Model file for the job. Use its own axes, mm. A direction names the side the tool comes from. Coordinates: 2 decimals unless noted, no trailing zeros. Write each loop counter-clockwise with the first axis right and the second up, starting at its lowest first coordinate (ties: lowest second). Pieces come first, ordered by that corner, then holes. Notation, with made-up numbers: (84, 16.5) - (129, 16.5) arc R22 cw to (129, 45.5) - close; hole circle Ø8 at (36.5, 29). An arc over 180 degrees is marked (long way). Put each result on its own line as item: value. Start each with the question number.
1. Saw through at B-B, the plane y = 0.5. Write the cut outline in (x, z), plus the area to 3 significant figures.
2. Which spindle directions (+Z, -Z, +X, -X, +Y, -Y) get a long thin tool onto all of the face, cutting with end or side? Do faces 3 (the face through (0, 1, 2.5)), 4 (the face through (22, 2, 1)). Say none if no direction does.
3. Drill centre lines: L1, parallel to X at y = 1.5, z = 0; L2, parallel to X at y = 2.7, z = 0; L3, parallel to Y at x = -14, z = -0.3. Where is each one in solid material? Low to high. Write a range as from..to.
4. Pull direction X, two halves, no side cores. Call faces 1 (the face through (21, 1, 0)), 2 (the face through (-24, 3, 0)): released by +X, released by -X, zero draft, split by the parting line, or undercut.
5. Saw through at A-A, the plane z = 0. Write the cut outline in (x, y), plus the area to 3 significant figures.
6. Drop a flat-ended pin along its axis: P1, Ø2.5, axis at x = 21.75, z = 0, coming from the +Y side. Give the stop position or say it passes through.
7. Saw through at C-C, the plane x = 11.5. Write the cut outline in (y, z), plus the area to 3 significant figures.
```python
from build123d import *
from build123d.topology import SkipClean

# Parameters (mm, degrees)
SKETCH2_R           = 0.75
BOSS_EXTRUDE1_DEPTH = 2
SKETCH3_R           = 2.5
SKETCH3_R_2         = 2
BOSS_EXTRUDE2_DEPTH = 1


with BuildPart() as part:
    # Sketch2 → Boss-Extrude1 (new body)
    with BuildSketch(Plane(origin=(0, 0, 0), x_dir=(1, 0, 0), z_dir=(0, 1, 0))):
        with BuildLine():
            Line((-21.75, 2.5), (21.75, 2.5))
            ThreePointArc((21.75, 2.5), (24.25, 0), (21.75, -2.5))
            Line((21.75, -2.5), (-21.75, -2.5))
            ThreePointArc((-21.75, -2.5), (-24.25, 0), (-21.75, 2.5))
        make_face()
        with Locations(Location((-21.75, 0, 0), (0, 0, 270))):
            Circle(SKETCH2_R, mode=Mode.SUBTRACT)
        with Locations(Location((21.75, 0, 0), (0, 0, 270))):
            Circle(SKETCH2_R, mode=Mode.SUBTRACT)
    extrude(amount=BOSS_EXTRUDE1_DEPTH)

    # Sketch3 → Boss-Extrude2 (add)
    # profile 1 of 2: a face of its own
    with SkipClean():  # the faces are left unmerged after this step: merging them gives an invalid solid
        with BuildSketch(Plane(origin=(0, 2, 0), x_dir=(1, 0, 0), z_dir=(0, 1, 0))):
            with Locations(Location((21.75, 0, 0), (0, 0, 270))):
                Circle(SKETCH3_R)
            with Locations(Location((21.75, 0, 0), (0, 0, 270))):
                Circle(SKETCH3_R_2, mode=Mode.SUBTRACT)
        # profile 2 of 2: a face of its own
        with BuildSketch(Plane(origin=(0, 2, 0), x_dir=(1, 0, 0), z_dir=(0, 1, 0))):
            with BuildLine():
                Line((-21.75, 2.5), (-21.75, 2))
                ThreePointArc((-21.75, 2), (-23.75, 0), (-21.75, -2))
                Line((-21.75, -2), (-21.75, -2.5))
                ThreePointArc((-21.75, -2.5), (-24.25, 0), (-21.75, 2.5))
            make_face()
        extrude(amount=BOSS_EXTRUDE2_DEPTH)
    add(part.part.scale(1), mode=Mode.REPLACE)  # the faces are merged on a copy


solid = part.part
```
Final values:
1. outline: (-21.75, -2.5) - (21.75, -2.5) arc R2.5 ccw to (21.75, 2.5) - (-21.75, 2.5) arc R2.5 ccw to start; hole circle Ø1.5 at (-21.75, 0); hole circle Ø1.5 at (21.75, 0)
1. area: 234 mm²
2. face 3: +Z, +X, -X, +Y, -Y
2. face 4: +Y
3. L1: x = -24.25..-22.5, -21..21, 22.5..24.25
3. L2: x = -24.25..-23.75, 19.25..19.75, 23.75..24.25
3. L3: y = 0..2
4. face 1: undercut
4. face 2: zero draft
5. outline: (-24.25, 0) - (-22.5, 0) - (-22.5, 2) - (-23.75, 2) - (-23.75, 3) - (-24.25, 3) - close; (-21, 0) - (21, 0) - (21, 2) - (19.75, 2) - (19.75, 3) - (19.25, 3) - (19.25, 2) - (-21, 2) - close; (22.5, 0) - (24.25, 0) - (24.25, 3) - (23.75, 3) - (23.75, 2) - (22.5, 2) - close
5. area: 92.5 mm²
6. P1: stops at y = 2
7. outline: (0, -2.5) - (2, -2.5) - (2, 2.5) - (0, 2.5) - close
7. area: 10.0 mm²
